Work out the finished part from the listing and answer in its coordinate system (mm). A direction names the side the tool comes from. Give positions to 0.01 mm unless a question says otherwise; leave off trailing zeros. Loops run counter-clockwise (first coordinate to the right, second up) from the corner with the lowest first, then second, coordinate; pieces in that order, holes last. Notation, with made-up numbers: (73, 54.25) - (110, 54.25) arc R23 ccw to (110, 79.25) - close; hole circle Ø2 at (-13.75, 10). An arc over 180 degrees is marked (long way). One line per question, with ' | ' between items.
from build123d import *

# Parameters (mm, degrees)
F1_DEPTH  = 75
F2_R      = 7.644408
F4_COUNT  = 6
F5_R      = 15
F6_DEPTH  = 11
F7_R      = 3.5
F7_R_2    = 0.95
F8_DEPTH  = 25
F10_DEPTH = 1
F11_R     = 2.5
F11_R_2   = 0.95
F12_DEPTH = 6


with BuildPart() as f1:
    # F0 (on Top) → F1 (new body)
    with BuildSketch(Plane.XY):
        Polygon((11.672223, -10.983332), (12, -10), (-3, 0), (-3.327777, -0.983332), align=None)
        Polygon((-3.327777, -0.983332), (-3, 0), (-6, 0), (-6, -0.983332), align=None)
    extrude(amount=-F1_DEPTH)

    # F2
    f2_edges = [f1.edges().sort_by_distance(p)[0] for p in [
        (-3.327777, -0.983332, -37.5),
        (-3, 0, -37.5),
    ]]
    fillet(f2_edges, radius=F2_R)



with BuildPart() as f4_1:
    # F4: instance of F1
    add(f1.part.rotate(Axis((0, 13.525062, 0), (0, 1, 0)), 1 * 360 / F4_COUNT))


with BuildPart() as f4_2:
    # F4: instance of F1
    add(f1.part.rotate(Axis((0, 13.525062, 0), (0, 1, 0)), 2 * 360 / F4_COUNT))


with BuildPart() as f4_3:
    # F4: instance of F1
    add(f1.part.rotate(Axis((0, 13.525062, 0), (0, 1, 0)), 3 * 360 / F4_COUNT))


with BuildPart() as f4_4:
    # F4: instance of F1
    add(f1.part.rotate(Axis((0, 13.525062, 0), (0, 1, 0)), 4 * 360 / F4_COUNT))


with BuildPart() as f4_5:
    # F4: instance of F1
    add(f1.part.rotate(Axis((0, 13.525062, 0), (0, 1, 0)), 5 * 360 / F4_COUNT))


with BuildPart() as f1_1:
    add(f1.part)

    add(f4_1.part)  # F6 merges F4_1

    add(f4_2.part)  # F6 merges F4_2

    add(f4_3.part)  # F6 merges F4_3

    add(f4_4.part)  # F6 merges F4_4

    add(f4_5.part)  # F6 merges F4_5
    # F5 (on Front) → F6 (join)
    with BuildSketch(Plane.XZ):
        Circle(F5_R)
    extrude(amount=F6_DEPTH)

    # F7 (on face) → F8 (cut)
    with BuildSketch(Plane(origin=(0, 0, 0), x_dir=(-1, 0, 0), z_dir=(0, 1, 0))):
        with Locations((-4.702282, 6.472136)):
            Circle(F7_R)
        with Locations((-7.608452, -2.472136)):
            Circle(F7_R)
        with Locations((0, -8)):
            Circle(F7_R)
        with Locations((7.608452, -2.472136)):
            Circle(F7_R)
        with Locations((4.702282, 6.472136)):
            Circle(F7_R)
        Circle(F7_R_2)
    extrude(amount=-F8_DEPTH, mode=Mode.SUBTRACT)

    # F9 (on face) → F10 (cut)
    with BuildSketch(Plane(origin=(0, 0, 0), x_dir=(-1, 0, 0), z_dir=(0, 1, 0))):
        with BuildLine():
            ThreePointArc((5.158171, -12.103592), (-1.067262, -13.113528), (-7.047458, -11.110221))
            Line((-7.047458, -11.110221), (-7.288358, -11.549476))
            ThreePointArc((-7.288358, -11.549476), (-1.091943, -13.613164), (5.354197, -12.563564))
            Line((5.354197, -12.563564), (5.746248, -13.483508))
            Line((5.746248, -13.483508), (7.096071, -11.549476))
            Line((7.096071, -11.549476), (4.76612, -11.183649))
            Line((4.76612, -11.183649), (5.158171, -12.103592))
        make_face()
        with BuildLine():
            Line((8.803936, 11.71815), (6.454104, 11.920116))
            Line((6.454104, 11.920116), (7.302264, 9.719405))
            Line((7.302264, 9.719405), (7.902933, 10.518903))
            ThreePointArc((7.902933, 10.518903), (11.89028, 5.632489), (13.145463, -0.548167))
            Line((13.145463, -0.548167), (13.646319, -0.537165))
            ThreePointArc((13.646319, -0.537165), (12.335317, 5.860932), (8.203267, 10.918652))
            Line((8.203267, 10.918652), (8.803936, 11.71815))
        make_face()
        with BuildLine():
            Line((-14.550184, 1.765357), (-13.550175, -0.370639))
            Line((-13.550175, -0.370639), (-12.068384, 1.464243))
            Line((-12.068384, 1.464243), (-13.061104, 1.584689))
            ThreePointArc((-13.061104, 1.584689), (-10.823018, 7.48104), (-6.098005, 11.658388))
            Line((-6.098005, 11.658388), (-6.357961, 12.086641))
            ThreePointArc((-6.357961, 12.086641), (-11.243374, 7.752232), (-13.557464, 1.644912))
            Line((-13.557464, 1.644912), (-14.550184, 1.765357))
        make_face()
    extrude(amount=-F10_DEPTH, mode=Mode.SUBTRACT)

    # F11 (on face) → F12 (join)
    with BuildSketch(Plane(origin=(0, 0, 0), x_dir=(-1, 0, 0), z_dir=(0, 1, 0))):
        Circle(F11_R)
        Circle(F11_R_2, mode=Mode.SUBTRACT)
    extrude(amount=F12_DEPTH)


solid = f1_1.part
1. Flat-ended cylindrical pins translate along their axes: pin 1 (15.5 mm diameter, centred on x = 24, z = -29.5, fed in from -Y); pin 2 (15.5 mm diameter, centred on x = -26, z = 28.5, fed in from -Y); pin 3 (1 mm diameter, centred on y = -2, z = -48.5, fed in from +X); pin 4 (1.1 mm diameter, centred on x = 0, z = 0, fed in from -Y). Find the tip coordinate at first contact, or state that the pin passes through.
Evaluation:
pin 1: y = -0.98 | pin 2: y = -1.18 | pin 3: x = 0.75 | pin 4: through
2. Find section B-B on y = 2.5. Write down the section's boundary in (x, z), then the cut area to 3 significant figures.
Evaluation:
outline: circle Ø5 at (0, 0); hole circle Ø1.9 at (0, 0) | area: 16.8 mm2
3. Which of the six approach directions +Z, -Z, +X, -X, +Y, -Y give full straight-line access (tool end or side, diameter ignored) to faces 4 (the cylindrical face through (11.19, -0.49, 7.83)), 5 (the flat face through (41.89, -10.5, -10.52)), 6 (the flat face through (-3, -5, 75)), 7 (the cylindrical face through (-3.069, -0.337, -44.94)), 8 (the cylindrical face through (-4.11, -5.42, -2.32))?
Evaluation:
face 4: +Y | face 5: +X, -Y | face 6: +Z, +X, -X, +Y, -Y | face 7: -Z, +Y | face 8: +Y, -Y
4. Determine the mould class of faces 1 (the cylindrical face through (-40.454, -0.337, -19.812)), 2 (the flat face through (40.97, -0.983, 16.93)), 3 (the cylindrical face through (-37.136, -1.302, 25.432)) for opening direction Z: +Z half, -Z half, draft (parallel to the pull), parting line (faces both ways), or undercut.
Evaluation:
face 1: -Z half | face 2: undercut | face 3: +Z half
5. Consider L1, parallel to Z at x = 0, y = 3.05; L2, parallel to Z at x = -6, y = -8; L3, parallel to Z at x = 22, y = -4. Determine where each line is inside the solid, lowest interval first.
Evaluation:
L1: -2.5 to -0.95, 0.95 to 2.5 | L2: -13.86 to -5.58, 0.64 to 3.22, 9.72 to 13.75 | L3: -11.32 to -9.24, 14.08 to 16.17
6. Find section C-C on z = 19. State how many separate pieces and enclosed holes the cut face has, then the cut area to 3 significant figures.
Evaluation:
separate pieces: 3 | enclosed holes: 0 | area: 104 mm2
7. Find section A-A on z = 45.5. Write down the section's boundary in (x, y), then the cut area to 3 significant figures.
Evaluation:
outline: (-12, -10) - (-11.67, -10.98) - (1.4, -2.27) arc R7.64 cw to (5.64, -0.98) - (6, -0.98) - (6, 0) - (5.31, 0) arc R7.64 ccw to (1.07, -1.28) - close; (54.81, -10) - (55.46, -10.98) - (60.33, -9.36) - (60.33, -8.16) - close | area: 27.1 mm2
